```python
from build123d import *

# Parameters (mm, degrees)
SKETCH_1_W          = 42
SKETCH_1_H          = 11
SKETCH_1_R          = 1.6
EXTRUDE_1_DEPTH     = 18
FILLET_1_R          = 3
SKETCH_3_R          = 3.5
CUT_EXTRUDE_2_DEPTH = 4
SKETCH_4_R          = 1.6
CUT_EXTRUDE_3_DEPTH = 11
CUT_EXTRUDE_4_DEPTH = 3


with BuildPart() as part:
    # 스케치1 → 보스-돌출1 (new body)
    with BuildSketch(Plane(origin=(0, -13.749164409, 0), x_dir=(1, 0, 0), z_dir=(0, 1, 0))):
        with Locations((-11.155757596, -57.302460642)):
            Rectangle(SKETCH_1_W, SKETCH_1_H)
        with Locations((-26.655757596, -57.302460642)):
            Circle(SKETCH_1_R, mode=Mode.SUBTRACT)
        with Locations((4.344242404, -57.302460642)):
            Circle(SKETCH_1_R, mode=Mode.SUBTRACT)
    extrude(amount=EXTRUDE_1_DEPTH)

    # 필렛1
    fillet_1_edges = [part.edges().sort_by_distance(p)[0] for p in [
        (-32.155757596, -4.749164409, 51.802460642),
        (9.844242404, -4.749164409, 51.802460642),
        (9.844242404, -4.749164409, 62.802460642),
        (-32.155757596, -4.749164409, 62.802460642),
    ]]
    fillet(fillet_1_edges, radius=FILLET_1_R)

    # 스케치3 → 컷-돌출2 (cut)
    with BuildSketch(Plane(origin=(0, 4.250835591, 0), x_dir=(1, 0, 0), z_dir=(0, 1, 0))):
        with Locations((-26.655757596, -57.302460642)):
            Circle(SKETCH_3_R)
        with Locations((4.344242404, -57.302460642)):
            Circle(SKETCH_3_R)
    extrude(amount=-CUT_EXTRUDE_2_DEPTH, mode=Mode.SUBTRACT)

    # 스케치4 → 컷-돌출3 (cut)
    with BuildSketch(Plane(origin=(0, 0, 51.802460642), x_dir=(-1, 0, 0), z_dir=(0, 0, -1))):
        with Locations((11.155757596, -1.249164409)):
            Circle(SKETCH_4_R)
        with Locations((11.155757596, -8.249164409)):
            Circle(SKETCH_4_R)
    extrude(amount=-CUT_EXTRUDE_3_DEPTH, mode=Mode.SUBTRACT)

    # 스케치6 → 컷-돌출4 (cut)
    with BuildSketch(Plane.XY.offset(62.802460642)):
        Polygon((-7.922596089, -1.249164409), (-9.539176842, 1.550835591), (-12.77233835, 1.550835591), (-14.388919104, -1.249164409), (-12.77233835, -4.049164409), (-9.539176842, -4.049164409), align=None)
        Polygon((-7.922596089, -8.249164409), (-9.539176842, -5.449164409), (-12.77233835, -5.449164409), (-14.388919104, -8.249164409), (-12.77233835, -11.049164409), (-9.539176842, -11.049164409), align=None)
    extrude(amount=-CUT_EXTRUDE_4_DEPTH, mode=Mode.SUBTRACT)


solid = part.part
```
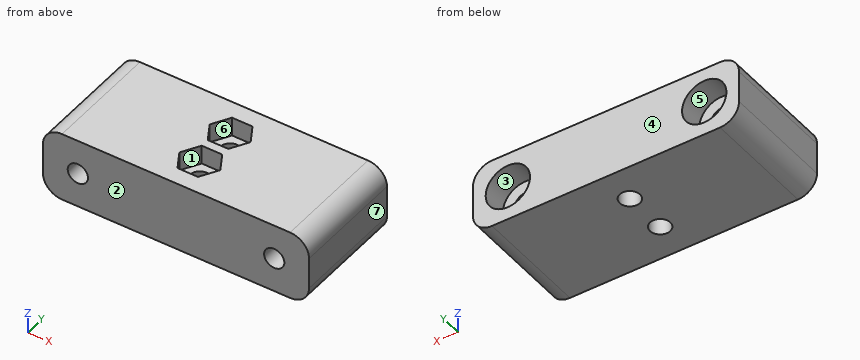
The model under review builds one solid part; all positions refer to its coordinate system, in mm. Face numbers are marked on the shaded views. A direction names the side the tool comes from. Round coordinates to 2 decimals unless told otherwise and drop trailing zeros. Loops run counter-clockwise (first coordinate to the right, second up) from the corner with the lowest first, then second, coordinate; pieces in that order, holes last. Notation, with made-up numbers: (25.5, 16.25) - (80.5, 16.25) arc R33 cw to (80.5, 51.25) - close; hole circle Ø4 at (13, -22.5). An arc over 180 degrees is marked (long way). Use a Markdown table: item, result. Add a question column.
Q1. Insertion check: pin 1 Ø1.5 at (y, z) = (1.5, 61) entering from +X; pin 2 Ø3.5 at (x, z) = (-27, 56) entering from +Y; pin 3 Ø3 at (x, y) = (-11.5, -7.5) entering from +Z. Each pin has a flat end and moves straight along its axis. Give the tip position at first contact, or say it passes through.
Q2. Machinability: for the marked faces 5, 6 and 7, which of the approach directions +Z, -Z, +X, -X, +Y, -Y give a long, thin tool a straight path to every point of the face, cutting with its end or side? Answer none if there is none.
Q3. Add section A-A (z = 56.75). State the section outline as (x, y) points.
Q4. Add section C-C (x = 4). State the section outline as (y, z) points, plus the area to 3 significant figures.
Q5. Add section D-D (z = 60.25). State the section outline as (x, y) points.
Q6. For probe 1 along X at (y, z) = (-12, 57.25); probe 2 along X at (y, z) = (-12, 57); probe 3 along Y at (x, z) = (-24.5, 60), list the stretches that pass through material, from the lowest coordinate up.
Q7. Add section B-B (y = -8.75). State the section outline as (x, z) points, plus the area to 3 significant figures.
Q8. The part is to be moulded in two halves that separate along Y. For the marked faces 1, 2, 3 and 4, say which applies: pulls with the +Y half, pulls with the -Y half, needs draft (parallel to the pull), parting line crosses it, or undercut.
Worked answers:
| question | item | result |
|---|---|---|
| 1 | pin 1 | x = 9.81 |
| 1 | pin 2 | y = 0.25 |
| 1 | pin 3 | z = 59.8 |
| 2 | face 5 | +Y |
| 2 | face 6 | +Z |
| 2 | face 7 | +Z, -Z, +X, +Y, -Y |
| 3 | outline | (-32.16, -13.75) - (-28.16, -13.75) - (-28.16, 0.25) - (-30.11, 0.25) - (-30.11, 4.25) - (-32.16, 4.25) - close; (-25.15, -13.75) - (2.84, -13.75) - (2.84, 0.25) - (0.89, 0.25) - (0.89, 4.25) - (-23.2, 4.25) - (-23.2, 0.25) - (-25.15, 0.25) - close; (5.85, -13.75) - (9.84, -13.75) - (9.84, 4.25) - (7.8, 4.25) - (7.8, 0.25) - (5.85, 0.25) - close; hole circle Ø3.2 at (-11.16, -8.25); hole circle Ø3.2 at (-11.16, -1.25) |
| 4 | outline | (-13.75, 51.8) - (4.25, 51.8) - (4.25, 53.82) - (0.25, 53.82) - (0.25, 55.74) - (-13.75, 55.74) - close; (-13.75, 58.86) - (0.25, 58.86) - (0.25, 60.79) - (4.25, 60.79) - (4.25, 62.8) - (-13.75, 62.8) - close |
| 4 | area | 126 mm² |
| 5 | outline | (-32.12, -13.75) - (9.81, -13.75) - (9.81, 4.25) - (6.23, 4.25) - (6.23, 0.25) - (2.46, 0.25) - (2.46, 4.25) - (-24.77, 4.25) - (-24.77, 0.25) - (-28.54, 0.25) - (-28.54, 4.25) - (-32.12, 4.25) - close; hole (-14.39, -8.25) - (-12.77, -11.05) - (-9.54, -11.05) - (-7.92, -8.25) - (-9.54, -5.45) - (-12.77, -5.45) - close; hole (-14.39, -1.25) - (-12.77, -4.05) - (-9.54, -4.05) - (-7.92, -1.25) - (-9.54, 1.55) - (-12.77, 1.55) - close |
| 6 | probe 1 | -32.16 to -28.25, -25.06 to 2.75, 5.94 to 9.84 |
| 6 | probe 2 | -32.16 to -28.23, -25.08 to 2.77, 5.92 to 9.84 |
| 6 | probe 3 | -13.75 to 0.25 |
| 7 | outline | (-32.16, 54.8) arc R3 ccw to (-29.16, 51.8) - (-12.68, 51.8) - (-12.68, 59.8) - (-14.1, 59.8) - (-14.1, 62.8) - (-29.16, 62.8) arc R3 ccw to (-32.16, 59.8) - close; (-9.64, 51.8) - (6.84, 51.8) arc R3 ccw to (9.84, 54.8) - (9.84, 59.8) arc R3 ccw to (6.84, 62.8) - (-8.21, 62.8) - (-8.21, 59.8) - (-9.64, 59.8) - close; hole circle Ø3.2 at (-26.66, 57.3); hole circle Ø3.2 at (4.34, 57.3) |
| 7 | area | 396 mm² |
| 8 | face 1 | undercut |
| 8 | face 2 | pulls with the -Y half |
| 8 | face 3 | needs draft |
| 8 | face 4 | pulls with the +Y half |
